from build123d import *

# Parameters (mm, degrees)
F0_R     = 7.49
F1_DEPTH = 22.5
F2_R     = 4
F3_DEPTH = 27.5


with BuildPart() as f1:
    # F0 (on Front) → F1 (new body, symmetric)
    with BuildSketch(Plane.XZ):
        Circle(F0_R)
    extrude(amount=F1_DEPTH, both=True)

    # F2 (on Front) → F3 (join, symmetric)
    with BuildSketch(Plane.XZ):
        Circle(F2_R)
    extrude(amount=F3_DEPTH, both=True)


solid = f1.part
Input: part model. Units: mm. Frame: model coordinates. A direction names the side the tool comes from. Coordinates: 2 decimals unless noted, no trailing zeros. Loops run counter-clockwise (first coordinate to the right, second up) from the corner with the lowest first, then second, coordinate; pieces in that order, holes last.
Q1. Cut plane D-D (x = -5). Output: boundary loops of the cut face in (y, z), then the cut area to 3 significant figures.
Q2. Material intervals for line 1 (Y direction, x = -4.75, z = -3.75); line 2 (X direction, y = -2.5, z = -3.25); line 3 (Z direction, x = -1, y = -24), sorted ascending.
Q3. Cut plane A-A (z = 0). Output: boundary loops of the cut face in (x, y).
Q4. Contact query for flat-ended pins moving along their axis: pin 1 (2 mm diameter, centred on y = 9.5, z = 4.5, fed in from -X); pin 2 (1 mm diameter, centred on x = -6, z = 0.5, fed in from -Y); pin 3 (1 mm diameter, centred on x = 3, y = 18, fed in from -Z). Output: stop coordinate, or through.
Q5. Set-up query: faces 1 (the face through (-0.867, 24.965, -3.905)), 2 (the face through (-0.867, -25.035, -3.905)), 3 (the face through (0, 27.5, 0)). Return all of +Z, -Z, +X, -X, +Y, -Y with unobstructed straight access to the full face (end or side cutting, diameter ignored); none if empty.
Q6. Cut plane B-B (x = 0). Output: boundary loops of the cut face in (y, z), then the cut area to 3 significant figures.
Q7. Cut plane C-C (y = 11). Output: boundary loops of the cut face in (x, z), then the cut area to 3 significant figures.
Working result:
1. outline: (-22.5, -5.58) - (22.5, -5.58) - (22.5, 5.58) - (-22.5, 5.58) - close
1. area: 502 mm2
2. line 1: y = -22.5 to 22.5
2. line 2: x = -6.75 to 6.75
2. line 3: z = -3.87 to 3.87
3. outline: (-7.49, -22.5) - (-4, -22.5) - (-4, -27.5) - (4, -27.5) - (4, -22.5) - (7.49, -22.5) - (7.49, 22.5) - (4, 22.5) - (4, 27.5) - (-4, 27.5) - (-4, 22.5) - (-7.49, 22.5) - close
4. pin 1: stops at x = -6.62
4. pin 2: stops at y = -22.5
4. pin 3: stops at z = -7.06
5. face 1: +Y
5. face 2: -Y
5. face 3: +Z, -Z, +X, -X, +Y
6. outline: (-27.5, -4) - (-22.5, -4) - (-22.5, -7.49) - (22.5, -7.49) - (22.5, -4) - (27.5, -4) - (27.5, 4) - (22.5, 4) - (22.5, 7.49) - (-22.5, 7.49) - (-22.5, 4) - (-27.5, 4) - close
6. area: 754 mm2
7. outline: circle Ø14.98 at (0, 0)
7. area: 176 mm2
